Autodesk Inventor part; units mm, degrees
ref_plane "YZ Plane" through (0, 0, 0) normal (1, 0, 0) x (0, 1, 0)
ref_plane "XZ Plane" through (0, 0, 0) normal (0, 1, 0) x (-1, 0, 0)
ref_plane "XY Plane" through (0, 0, 0) normal (0, 0, 1) x (1, 0, 0)
sketch "スケッチ3" plane through (0, 0, 0) normal (0, 0, 1) x (1, 0, 0)
  line L0 (129.999999, 177.723921) -> (129.999999, 194.723921)
  line L1 (129.999999, 194.723921) -> (-0.000001, 194.723921)
  line L2 (-0.000001, 0) -> (129.999999, 0)
  circle A0 centre (77.999999, 186.723921) radius 2.15
  circle A1 centre (91.999999, 186.723921) radius 2.15
  circle A2 centre (51.999999, 186.723921) radius 2.15
  circle A3 centre (37.999999, 186.723921) radius 2.15
  circle A4 centre (77.999999, 8) radius 2.15
  circle A5 centre (91.999999, 8) radius 2.15
  circle A6 centre (51.999999, 8) radius 2.15
  circle A7 centre (37.999999, 8) radius 2.15
  line L3 (129.999999, 129.723921) -> (19.999999, 129.723921)
  line L4 (13.999999, 135.723921) -> (13.999999, 177.723921)
  line L5 (13.999999, 177.723921) -> (129.999999, 177.723921)
  line L6 (19.999999, 129.723921) -> (13.999999, 135.723921)
  circle A8 centre (64.999999, 97.36196) radius 8
  circle A9 centre (7.999999, 186.723921) radius 1.6
  circle A10 centre (121.999999, 186.723921) radius 1.6
  circle A11 centre (121.999999, 8) radius 1.6
  circle A12 centre (7.999999, 8) radius 1.6
  circle A13 centre (7.999999, 82) radius 1.6
  circle A14 centre (121.999999, 82) radius 1.6
  line L7 (64.999999, 88.36196) -> (64.999999, 42.36196)
  line L8 (3.399999, 186.723921) -> (12.599999, 186.723921)
  line L9 (7.999999, 182.123921) -> (7.999999, 191.323921)
  line L10 (117.399999, 186.723921) -> (126.599999, 186.723921)
  line L11 (121.999999, 182.123921) -> (121.999999, 191.323921)
  line L12 (117.399999, 8) -> (126.599999, 8)
  line L13 (121.999999, 3.4) -> (121.999999, 12.6)
  line L14 (3.399999, 8) -> (12.599999, 8)
  line L15 (7.999999, 3.4) -> (7.999999, 12.6)
  line L16 (3.399999, 82) -> (12.599999, 82)
  line L17 (7.999999, 77.4) -> (7.999999, 86.6)
  line L18 (126.599999, 82) -> (117.399999, 82)
  line L19 (121.999999, 77.4) -> (121.999999, 86.6)
  circle A15 centre (91.999999, 186.723921) radius 2.15
  circle A16 centre (77.999999, 186.723921) radius 2.15
  circle A17 centre (51.999999, 186.723921) radius 2.15
  circle A18 centre (37.999999, 186.723921) radius 2.15
  circle A19 centre (64.999999, 97.36196) radius 8
  circle A20 centre (91.999999, 8) radius 2.15
  circle A21 centre (77.999999, 8) radius 2.15
  circle A22 centre (51.999999, 8) radius 2.15
  circle A23 centre (37.999999, 8) radius 2.15
  circle A24 centre (7.999999, 8) radius 1.6
  circle A25 centre (121.999999, 8) radius 1.6
  circle A26 centre (121.999999, 82) radius 1.6
  circle A27 centre (121.999999, 186.723921) radius 1.6
  circle A28 centre (7.999999, 186.723921) radius 1.6
  circle A29 centre (7.999999, 82) radius 1.6
  line L20 (-0.000001, 0) -> (129.999999, 0)
  line L21 (129.999999, 177.723921) -> (129.999999, 194.723921)
  line L22 (129.999999, 194.723921) -> (-0.000001, 194.723921)
  line L23 (129.999999, 177.723921) -> (13.999999, 177.723921)
  line L24 (13.999999, 177.723921) -> (13.999999, 135.723921)
  line L25 (13.999999, 135.723921) -> (19.999999, 129.723921)
  line L26 (-0.000001, 194.723921) -> (-0.000001, 119.36196)
  line L27 (-0.000001, 86.6) -> (-0.000001, 0)
  line L28 (-0.000001, 194.723921) -> (-0.000001, 119.36196)
  line L29 (-0.000001, 86.6) -> (-0.000001, 0)
  line L30 (129.999999, 0) -> (129.999999, 86.6)
  line L31 (129.999999, 125.36196) -> (129.999999, 129.723921)
  line L32 (129.999999, 0) -> (129.999999, 86.6)
  line L33 (129.999999, 125.36196) -> (129.999999, 129.723921)
  circle A30 centre (18.296419, 23) radius 1.6
  circle A31 centre (111.703579, 23) radius 1.6
  line L34 (-0.000001, 119.36196) -> (-0.000001, 86.6)
  line L35 (129.999999, 86.6) -> (129.999999, 125.36196)
  point P0 (0, 0)
  point P1 (0, 0)
sketch "スケッチ4" plane through (0, 0, 0) normal (0, 0, 1) x (1, 0, 0)
  point P0 (0, 0)
extrude "押し出し1" add sketch "スケッチ3" along normal blind 4 contours L5 L4 L6 L3 L31 L35 L30 L2 L27 L34 L26 L1 L0 | A30 | A31
sketch "スケッチ5" plane through (0, 0, 4) normal (0, 0, 1) x (1, 0, 0)
  line L0 (-10, 0) -> (140, 0)
  arc A0 (140, -0.0003) -> (140, 0.0003) centre (140, 0) ccw
  arc A1 (-10, 0.0003) -> (-10, -0.0003) centre (-10, 0) ccw
  line L1 (140, 0) -> (140, 194.7239)
  arc A2 (140.0002, 194.7239) -> (139.9998, 194.7239) centre (140, 194.7239) ccw
  arc A3 (139.9998, 0) -> (140.0002, 0) centre (140, 0) ccw
  line L2 (140, 194.7239) -> (-10, 194.7239)
  arc A4 (-10, 194.7242) -> (-10, 194.7237) centre (-10, 194.72395) ccw
  arc A5 (140, 194.7237) -> (140, 194.7242) centre (140, 194.72395) ccw
  arc A6 (-10.0004, 0) -> (-10, 0) centre (-10.0002, 0) ccw
  arc A7 (-9.9996, 194.7239) -> (-10, 194.7239) centre (-9.9998, 194.7239) ccw
  arc A8 (65, 88.362) -> (65, 106.362) centre (65, 97.362) ccw
  arc A9 (65, 106.362) -> (65, 88.362) centre (65, 97.362) ccw
  arc A10 (65, 158.7239) -> (65, 176.7239) centre (65, 167.7239) ccw
  arc A11 (65, 176.7239) -> (65, 158.7239) centre (65, 167.7239) ccw
  line L3 (125.6971, 165.1236) -> (118.0771, 165.1236)
  line L4 (115.5371, 165.1236) -> (115.5371, 160.0436)
  line L5 (121.66, 165.205) -> (120.39, 165.205)
  arc A12 (121.66, 165.1669) -> (121.66, 165.2431) centre (121.66, 165.205) ccw
  line L6 (81.02, 174.095) -> (85.719, 174.095)
  arc A13 (81.02, 174.1331) -> (81.02, 174.0569) centre (81.02, 174.095) ccw
  line L7 (81.02, 174.095) -> (81.02, 165.205)
  arc A14 (80.9819, 165.205) -> (81.0581, 165.205) centre (81.02, 165.205) ccw
  arc A15 (81.0581, 174.095) -> (80.9819, 174.095) centre (81.02, 174.095) ccw
  line L8 (121.66, 165.205) -> (121.66, 174.095)
  arc A16 (121.6981, 174.095) -> (121.6219, 174.095) centre (121.66, 174.095) ccw
  arc A17 (121.6219, 165.205) -> (121.6981, 165.205) centre (121.66, 165.205) ccw
  line L9 (82.29, 165.205) -> (81.02, 165.205)
  arc A18 (81.02, 165.2431) -> (81.02, 165.1669) centre (81.02, 165.205) ccw
  line L10 (121.66, 174.095) -> (117.342, 174.095)
  arc A19 (121.66, 174.0569) -> (121.66, 174.1331) centre (121.66, 174.095) ccw
  line L11 (52.85, 166.325) -> (48.151, 166.325)
  arc A20 (52.85, 166.2869) -> (52.85, 166.3631) centre (52.85, 166.325) ccw
  line L12 (52.85, 166.325) -> (52.85, 175.215)
  arc A21 (52.8881, 175.215) -> (52.8119, 175.215) centre (52.85, 175.215) ccw
  arc A22 (52.8119, 166.325) -> (52.8881, 166.325) centre (52.85, 166.325) ccw
  line L13 (51.58, 175.215) -> (52.85, 175.215)
  arc A23 (52.85, 175.1769) -> (52.85, 175.2531) centre (52.85, 175.215) ccw
  arc A24 (72.9742, 175.4632) -> (72.9742, 175.768) centre (72.9742, 175.6156) ccw
  arc A25 (72.9742, 175.768) -> (72.9742, 175.4632) centre (72.9742, 175.6156) ccw
  arc A26 (72.9742, 175.4632) -> (72.9742, 175.768) centre (72.9742, 175.6156) ccw
  arc A27 (72.9742, 175.768) -> (72.9742, 175.4632) centre (72.9742, 175.6156) ccw
  arc A28 (86.106, 110.5662) -> (86.106, 110.871) centre (86.106, 110.7186) ccw
  arc A29 (86.106, 110.871) -> (86.106, 110.5662) centre (86.106, 110.7186) ccw
  arc A30 (86.106, 110.5662) -> (86.106, 110.871) centre (86.106, 110.7186) ccw
  arc A31 (86.106, 110.871) -> (86.106, 110.5662) centre (86.106, 110.7186) ccw
  line L14 (80.9819, 174.095) -> (121.6981, 174.095)
  line L15 (121.6981, 174.095) -> (121.6981, 165.205)
  line L16 (121.6981, 165.205) -> (80.9819, 165.205)
  line L17 (80.9819, 165.205) -> (80.9819, 174.095)
  line L18 (52.8, 176.585002) -> (11.364013, 176.585002)
  line L19 (11.364013, 176.585002) -> (11.364013, 165.1236)
  line L20 (11.364013, 165.1236) -> (52.8, 165.1236)
  line L21 (52.8, 165.1236) -> (52.8, 176.585002)
  line L22 (-10, 194.7239) -> (-10, 0)
  line L23 (21.97, 192.403451) -> (33.97, 192.403451)
  line L24 (33.97, 192.403451) -> (33.97, 183.403451)
  line L25 (33.97, 183.403451) -> (21.97, 183.403451)
  line L26 (21.97, 183.403451) -> (21.97, 192.403451)
  line L27 (0, 0) -> (129.999999, 0)
  line L28 (96.51585, 13.395653) -> (107.51585, 13.395653)
  line L29 (107.51585, 13.395653) -> (107.51585, 4.395653)
  line L30 (107.51585, 4.395653) -> (96.51585, 4.395653)
  line L31 (96.51585, 4.395653) -> (96.51585, 13.395653)
  circle A32 centre (65, 97.362) radius 9
  point P0 (71.80055, 0)
sketch "スケッチ5 outline for 押し出し2" plane through (0, 0, 4) normal (0, 0, 1) x (1, 0, 0)
  line L0 (96.51585, 13.395653) -> (107.51585, 13.395653)
  line L1 (107.51585, 13.395653) -> (107.51585, 4.395653)
  line L2 (107.51585, 4.395653) -> (96.51585, 4.395653)
  line L3 (96.51585, 4.395653) -> (96.51585, 13.395653)
  line L4 (21.97, 192.403451) -> (33.97, 192.403451)
  line L5 (33.97, 192.403451) -> (33.97, 183.403451)
  line L6 (33.97, 183.403451) -> (21.97, 183.403451)
  line L7 (21.97, 183.403451) -> (21.97, 192.403451)
  circle A0 centre (65, 97.362) radius 9
  line L8 (121.6981, 165.205) -> (121.6981, 174.095)
  line L9 (80.9819, 165.205) -> (121.6981, 165.205)
  line L10 (80.9819, 174.095) -> (80.9819, 165.205)
  line L11 (121.6981, 174.095) -> (80.9819, 174.095)
extrude "押し出し2" cut sketch "スケッチ5 outline for 押し出し2" against normal blind 10
sketch "スケッチ7" plane through (0, 0, 4) normal (0, 0, 1) x (1, 0, 0)
  point P0 (0, 0)
sketch "スケッチ8" plane through (0, 0, 4) normal (0, 0, 1) x (1, 0, 0)
  circle A0 centre (18.296419, 23) radius 1.6
  circle A1 centre (111.703579, 23) radius 1.6
  point P0 (0, 0)
extrude "押し出し5" cut sketch "スケッチ8" against normal blind 4
properties part number "2枚目kai" material "MDF 中密度繊維ボード"
Here's how the part is built. I have some questions about the finished solid (model axes, mm). A direction names the side the tool comes from. Give positions to 0.01 mm unless a question says otherwise; leave off trailing zeros. Order: outer loops, then holes, each group sorted by start corner. A loop starts at its lowest first (then second) coordinate and runs counter-clockwise, first axis right, second up. Notation, with made-up numbers: (-26, 26) -> (21, 26) arc R27 cw to (21, 50) -> close; hole circle Ø9 at (14.25, 56). An arc over 180 degrees is marked (long way). Use a Markdown table: item, result. Add a question column.
Item 1: For faces 4 (the face through (102, 13.396, 2)), 5 (the face through (66, 194.724, 2)), 6 (the face through (76, 129.724, 2)), which set-ups out of +Z, -Z, +X, -X, +Y, -Y let a thin tool reach every point of the face, with its end or its side?
Item 2: Will this pin go through, and if not, where does the flat tip stop? pin 1 (2.5 mm diameter, centred on x = 38, y = 186.72, fed in from -Z).
Item 3: Imagine slicing it at D-D on y = 162.5. Please give me the cut outline in (x, z).
Item 4: Imagine slicing it at A-A on x = 65. Please give me the cut outline in (y, z).
Item 5: If we mould it in two halves opening along Y, with no side actions, what happens to faces 1 (the face through (130, 64, 2)), 2 (the face through (64, 0, 2)), 3 (the face through (76.415, 6.547, 1.972))? For each: pulls with the +Y half, pulls with the -Y half, needs draft (parallel to the pull), parting line crosses it, or undercut.
Item 6: I need wall thicknesses on line 1 (Y direction, x = 78, z = 2.75); line 2 (Y direction, x = 25, z = 2.35); line 3 (X direction, y = 82, z = 1.45). Which ranges of each line are inside material? Lowest first, please.
Item 7: Imagine slicing it at B-B on x = 38. Please give me the cut outline in (y, z).
Item 8: Imagine slicing it at C-C on z = 0.7. Give the number of separate pieces and of enclosed holes in the cut face, plus the area to 3 significant figures.
Data:
| question | item | result |
|---|---|---|
| 1 | face 4 | +Z, -Z |
| 1 | face 5 | +Z, -Z, +X, -X, +Y |
| 1 | face 6 | +Z, -Z, +X |
| 2 | pin 1 | passes through |
| 3 | outline | (0, 0) -> (14, 0) -> (14, 4) -> (0, 4) -> close |
| 4 | outline | (0, 0) -> (88.36, 0) -> (88.36, 4) -> (0, 4) -> close; (106.36, 0) -> (129.72, 0) -> (129.72, 4) -> (106.36, 4) -> close; (177.72, 0) -> (194.72, 0) -> (194.72, 4) -> (177.72, 4) -> close |
| 5 | face 1 | needs draft |
| 5 | face 2 | pulls with the -Y half |
| 5 | face 3 | undercut |
| 6 | line 1 | y = 0 to 5.85, 10.15 to 129.72, 177.72 to 184.57, 188.87 to 194.72 |
| 6 | line 2 | y = 0 to 129.72, 177.72 to 183.4, 192.4 to 194.72 |
| 6 | line 3 | x = 0 to 6.4, 9.6 to 120.4, 123.6 to 130 |
| 7 | outline | (0, 0) -> (5.85, 0) -> (5.85, 4) -> (0, 4) -> close; (10.15, 0) -> (129.72, 0) -> (129.72, 4) -> (10.15, 4) -> close; (177.72, 0) -> (184.57, 0) -> (184.57, 4) -> (177.72, 4) -> close; (188.87, 0) -> (194.72, 0) -> (194.72, 4) -> (188.87, 4) -> close |
| 8 | separate pieces | 1 |
| 8 | enclosed holes | 19 |
| 8 | area | 19,100 mm² |
